Design review of the part built by this model. Coordinates are the model's own, in mm. Face numbers are marked on the shaded views. A direction names the side the tool comes from. Give positions to 0.01 mm unless a question says otherwise; leave off trailing zeros. Write each loop counter-clockwise with the first axis right and the second up, starting at its lowest first coordinate (ties: lowest second). Pieces come first, ordered by that corner, then holes. Notation, with made-up numbers: (19.25, 79.25) -> (50.25, 79.25) arc R7 cw to (50.25, 90.25) -> close; hole circle Ø2 at (86, -31). An arc over 180 degrees is marked (long way). Use CSV: the item, a comma, the result in double quotes.
```python
from build123d import *

# Parameters (mm, degrees)
F0_W     = 50.8
F0_H     = 25.4
F1_DEPTH = 25.4
F2_W     = 25.4
F2_H     = 25.4
F3_DEPTH = 50.8
F4_W     = 25.4
F4_H     = 25.4
F5_DEPTH = 25.4
F6_R     = 25.39999


# Not quite as in the source:
# - a fillet or chamfer is up to 0.001 mm smaller than in the source, because OpenCascade refuses the exact size


with BuildPart() as f1:
    # F0 (on Top) → F1 (new body)
    with BuildSketch(Plane.XY):
        with Locations((25.4, 12.7)):
            Rectangle(F0_W, F0_H)
    extrude(amount=F1_DEPTH)

    # F2 (on face) → F3 (join)
    with BuildSketch(Plane.XY.offset(25.4)):
        with Locations((12.7, 12.7)):
            Rectangle(F2_W, F2_H)
    extrude(amount=F3_DEPTH)

    # F4 (on face) → F5 (join)
    with BuildSketch(Plane(origin=(0, 0, 0), x_dir=(0, -1, 0), z_dir=(-1, 0, 0))):
        with Locations((-12.7, 63.5)):
            Rectangle(F4_W, F4_H)
    extrude(amount=F5_DEPTH)

    # F6 (radius 25.4 in the source; OpenCascade refuses exactly that, so slightly less here)
    f6_edges = [f1.edges().sort_by_distance(p)[0] for p in [
        (50.8, 12.7, 0),
        (-25.4, 12.7, 76.2),
    ]]
    fillet(f6_edges, radius=F6_R)


solid = f1.part
```
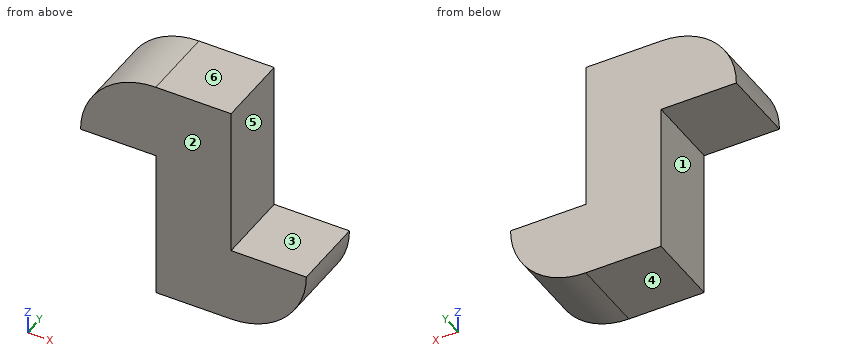
(1) Tool access review of the marked faces 1, 2 and 3: name each direction out of +Z, -Z, +X, -X, +Y, -Y from which nothing blocks a thin tool from reaching the whole face with its end or side.
Established:
face 1,"-Z, -X, +Y, -Y"
face 2,"+Z, -Z, +X, -X, -Y"
face 3,"+Z, +X, +Y, -Y"
(2) Take a section at B-B (z = 38.5). Write out the cut boundary in (x, y), then the cut area to 3 significant figures.
Established:
outline,"(0, 0) -> (25.4, 0) -> (25.4, 25.4) -> (0, 25.4) -> close"
area,"645 mm2"
(3) For line 1 along X through (y, z) = (1.5, 39); line 2 along X through (y, z) = (24.75, 51.5); line 3 along Z through (x, y) = (32.5, 9.25), list the stretches that pass through material, from the lowest coordinate up. Write a range as [from, to].
Established:
line 1,"x = [0, 25.4]"
line 2,"x = [-25.39, 25.4]"
line 3,"z = [1.01, 25.4]"
(4) Clearance check with flat-ended pins moving along their axes: pin 1 (12 mm diameter, centred on y = 11.5, z = 49, fed in from +X); pin 2 (4 mm diameter, centred on x = -9.5, z = 47, fed in from -Y); pin 3 (12.5 mm diameter, centred on x = 35, y = 8.5, fed in from +Z); pin 4 (2 mm diameter, centred on y = 17.5, z = 11, fed in from -X). State where each tip first meets the part, or that it passes through.
Established:
pin 1,"stops at x = 25.4"
pin 2,"passes through"
pin 3,"stops at z = 25.4"
pin 4,"stops at x = 0"
(5) Take a section at C-C (x = -7.5). Write out the cut boundary in (y, z).
Established:
outline,"(0, 50.8) -> (25.4, 50.8) -> (25.4, 75.07) -> (0, 75.07) -> close"
(6) Mouldability with a two-part tool opening along Z and no side actions: class the marked faces 4, 5 and 6 as +Z half, -Z half, draft (parallel to the pull), parting line (faces both ways), or undercut.
Established:
face 4,"-Z half"
face 5,"draft"
face 6,"+Z half"
